Design review of the part shown in the three views and the two pictorial views. Dimensions are in mm from the part's minimum x, y and z. Round coordinates to 2 decimals unless told otherwise and drop trailing zeros. Order: outer loops, then holes, each group sorted by start corner. A loop starts at its lowest first (then second) coordinate and runs counter-clockwise, first axis right, second up.
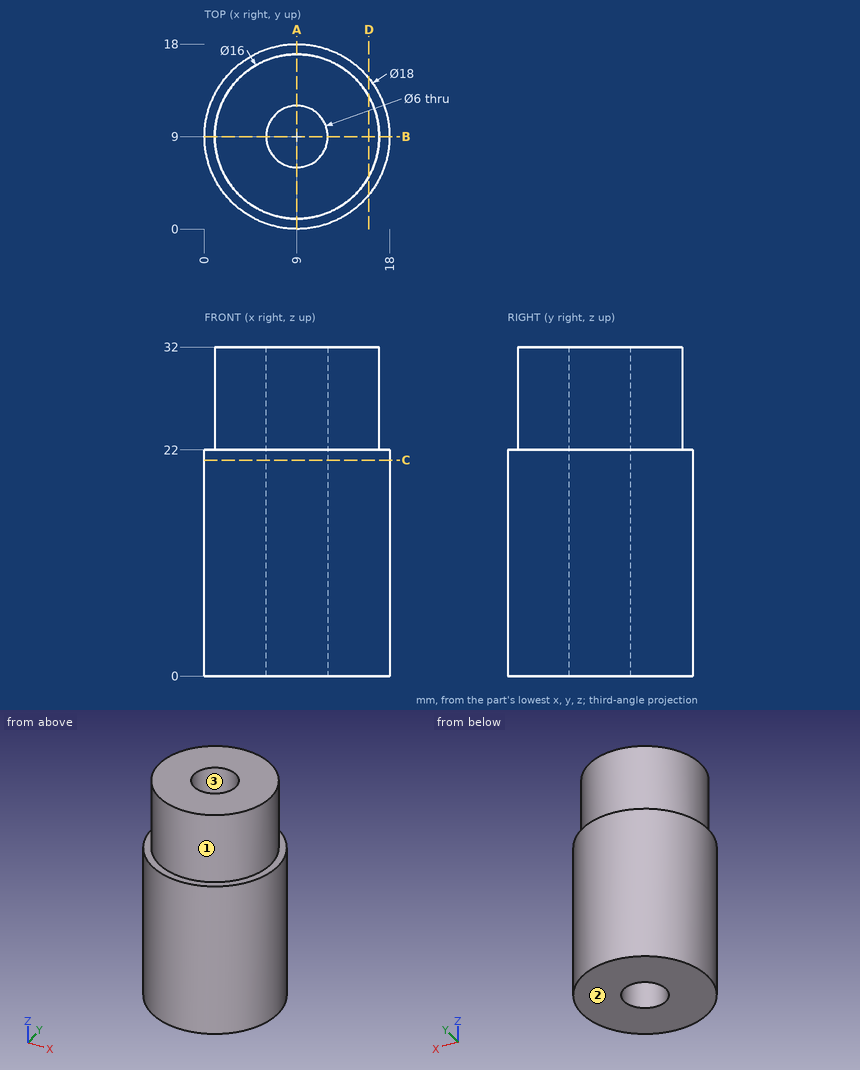
(1) Consider section D-D (x = 16). Write out the cut boundary in (y, z).
Data:
outline: (3.34, 0) - (14.66, 0) - (14.66, 22) - (12.87, 22) - (12.87, 32) - (5.13, 32) - (5.13, 22) - (3.34, 22) - close
(2) Consider section A-A (x = 9). Write out the cut boundary in (y, z), and give its area (3 significant figures).
Data:
outline: (0, 0) - (6, 0) - (6, 32) - (1, 32) - (1, 22) - (0, 22) - close; (12, 0) - (18, 0) - (18, 22) - (17, 22) - (17, 32) - (12, 32) - close
area: 364 mm2
(3) Insertion check: pin 1 (1 mm diameter, centred on x = 7.5, z = 5, fed in from -Y); pin 2 (5 mm diameter, centred on x = 16, z = 26, fed in from +Y); pin 3 (8 mm diameter, centred on x = 3.5, z = 11, fed in from +Y). Each pin has a flat end and moves straight along its axis. Give the tip position at first contact, or say it passes through.
Data:
pin 1: stops at y = 0.06
pin 2: stops at y = 15.61
pin 3: stops at y = 17.87
(4) Draft analysis for pull direction Y (two halves, no side actions). For the marked faces 1, 2 and 3, state which applies: pulls with the +Y half, pulls with the -Y half, needs draft (parallel to the pull), parting line crosses it, or undercut.
Data:
face 1: parting line crosses it
face 2: needs draft
face 3: undercut
(5) Consider section C-C (z = 21). Write out the cut boundary in (x, y), and give its area (3 significant figures).
Data:
outline: circle Ø18 at (9, 9); hole circle Ø6 at (9, 9)
area: 226 mm2
(6) To check wall thickness, follow probe 1 along Y at (x, z) = (9, 8.5); probe 2 along Y at (x, z) = (9, 24); probe 3 along Z at (x, y) = (4.25, 2.5). State the ranges of each line that lie inside material, in increasing order.
Data:
probe 1: y = 0 to 6, 12 to 18
probe 2: y = 1 to 6, 12 to 17
probe 3: z = 0 to 22
